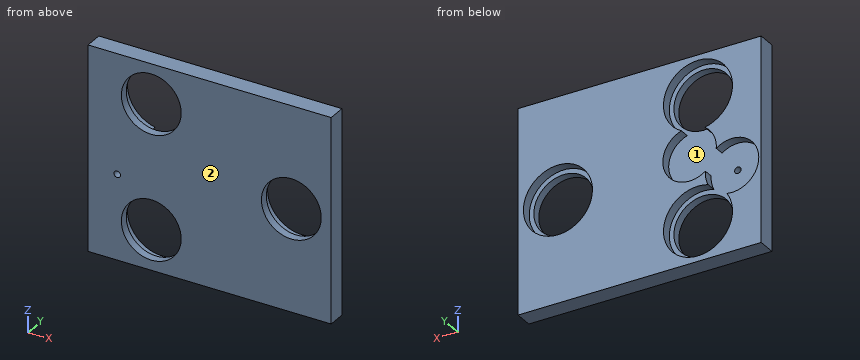
from build123d import *

# Parameters (mm, degrees)
SKETCH1_W                                      = 125
SKETCH1_H                                      = 105
TEST_BASE_POSTION_DEPTH                        = 9.215
THUMB_KNUCKLE_MOUNT_START                      = -4.215
SKETCH7_R                                      = 17.75
THUMB_KNUCKLE_MOUNT_DEPTH                      = 5
SKETCH8_R                                      = 15.375
THUMB_KNUCKLE_DEPTH                            = 4.215
GEARS_POSITION_EXTRUDE_CUT_START               = -4.215
SKETCH10_R                                     = 13.75
SKETCH10_R_2                                   = 17.75
GEARS_POSITION_EXTRUDE_CUT_DEPTH               = 5
SKETCH11_R                                     = 15.375
SKETCH11_R_2                                   = 1.65
FINGERS_KNUCKLE_MOUNT_AND_INTERMEDIATE_T_DEPTH = 83.142657767


with BuildPart() as part:
    # Sketch1 → Test_Base_Postion (new body)
    with BuildSketch(Plane(origin=(0, 0, 0), x_dir=(1, 0, 0), z_dir=(0, 1, 0))):
        Rectangle(SKETCH1_W, SKETCH1_H)
    extrude(amount=TEST_BASE_POSTION_DEPTH)

    # Sketch7 → Thumb_Knuckle_Mount (cut)
    with BuildSketch(Plane.XZ.offset(THUMB_KNUCKLE_MOUNT_START)):
        with Locations(Location((42, 0, 0), (0, 0, 270))):
            Circle(SKETCH7_R)
    extrude(amount=-THUMB_KNUCKLE_MOUNT_DEPTH, mode=Mode.SUBTRACT)

    # Sketch8 → Thumb_Knuckle (cut)
    with BuildSketch(Plane.XZ):
        with Locations(Location((42, 0, 0), (0, 0, 270))):
            Circle(SKETCH8_R)
    extrude(amount=-THUMB_KNUCKLE_DEPTH, mode=Mode.SUBTRACT)

    # Sketch10 → Gears_Position_Extrude_Cut (cut)
    with BuildSketch(Plane.XZ.offset(GEARS_POSITION_EXTRUDE_CUT_START)):
        with Locations((-25.678431211, 3.323807031)):
            Circle(SKETCH10_R)
        with Locations((-30, 32)):
            Circle(SKETCH10_R_2)
        with Locations((-47.5, -8.87533784)):
            Circle(SKETCH10_R)
        with Locations((-30, -32)):
            Circle(SKETCH10_R_2)
    extrude(amount=-GEARS_POSITION_EXTRUDE_CUT_DEPTH, mode=Mode.SUBTRACT)

    # Sketch11 → Fingers_Knuckle_Mount_and_Intermediate_Through_Hole (cut, through all)
    with BuildSketch(Plane.XZ):
        with Locations(Location((-30, 32, 0), (0, 0, 270))):
            Circle(SKETCH11_R)
        with Locations(Location((-30, -32, 0), (0, 0, 270))):
            Circle(SKETCH11_R)
        with Locations(Location((-47.5, -8.87533784, 0), (0, 0, 270))):
            Circle(SKETCH11_R_2)
    extrude(amount=-FINGERS_KNUCKLE_MOUNT_AND_INTERMEDIATE_T_DEPTH, mode=Mode.SUBTRACT)


solid = part.part
Geometry: final body of the model. Coordinates: model frame, mm. Face numbers are marked on the shaded views. Round coordinates to 2 decimals unless told otherwise and drop trailing zeros. Loops run counter-clockwise (first coordinate to the right, second up) from the corner with the lowest first, then second, coordinate; pieces in that order, holes last.
Q1. Section B-B on x = 42. Return loops of the section in (y, z) (3 decimals).
Q2. Pin query (flat end, axial travel): P1, Ø2, axis at x = -19, z = -19, coming from the -Y side; P2, Ø16.5, axis at x = -25.68, z = 3.32, coming from the +Y side (3 decimals). Return the tip coordinate at first contact, or that it passes through.
Q3. Material intervals for L1, parallel to X at y = 7.1, z = -32; L2, parallel to X at y = 7, z = -8.5; L3, parallel to Z at x = -25.5, y = 7.75, sorted ascending.
Q4. Pull-direction query (Z, two-part tool) for the marked faces 1 and 2; classes: released by +Z, released by -Z, zero draft, split by the parting line, or undercut.
Q5. Section C-C on z = -2. Return loops of the section in (x, y) (3 decimals), plus the area to 3 significant figures.
Q6. Section A-A on z = -32. Return loops of the section in (x, y) (3 decimals).
Evaluation:
1. outline: (0, -52.5) - (9.215, -52.5) - (9.215, -17.75) - (4.215, -17.75) - (4.215, -15.375) - (0, -15.375) - close; (0, 15.375) - (4.215, 15.375) - (4.215, 17.75) - (9.215, 17.75) - (9.215, 52.5) - (0, 52.5) - close
2. P1: stops at y = 0
2. P2: stops at y = 4.215
3. L1: x = -62.5 to -47.75, -12.25 to 62.5
3. L2: x = -62.5 to -61.24, -33.76 to -32.7, -18.66 to 26.42, 57.58 to 62.5
3. L3: z = -52.5 to -49.17, -14.83 to -10.43, 49.17 to 52.5
4. face 1: undercut
4. face 2: zero draft
5. outline: (-62.5, 0) - (26.756, 0) - (26.756, 4.215) - (24.363, 4.215) - (24.363, 9.215) - (-13.001, 9.215) - (-13.001, 4.215) - (-59.408, 4.215) - (-59.408, 9.215) - (-62.5, 9.215) - close; (57.244, 0) - (62.5, 0) - (62.5, 9.215) - (59.637, 9.215) - (59.637, 4.215) - (57.244, 4.215) - close
5. area: 615 mm2
6. outline: (-62.5, 0) - (-45.375, 0) - (-45.375, 4.215) - (-47.75, 4.215) - (-47.75, 9.215) - (-62.5, 9.215) - close; (-14.625, 0) - (62.5, 0) - (62.5, 9.215) - (-12.25, 9.215) - (-12.25, 4.215) - (-14.625, 4.215) - close
